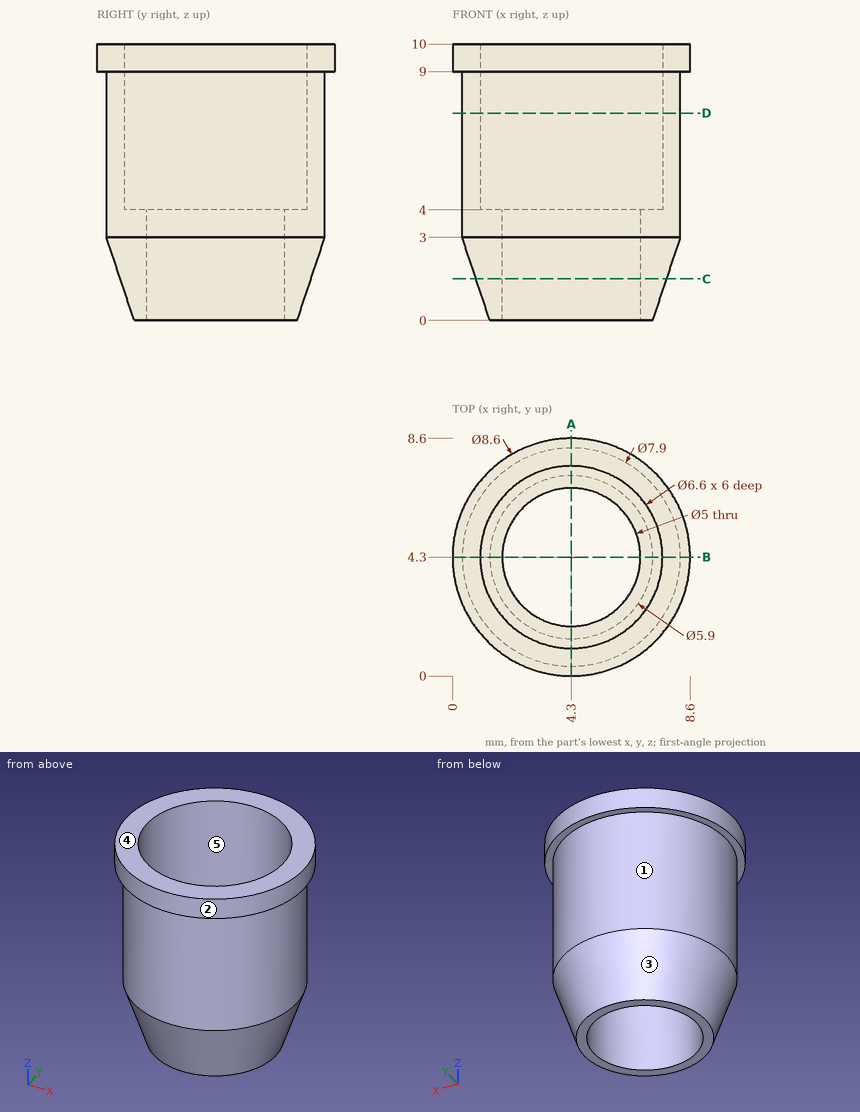
Print and shaded views of the part. All mm, measured from the part's lowest x, y and z. A direction names the side the tool comes from. Round coordinates to 2 decimals unless told otherwise and drop trailing zeros. Write each loop counter-clockwise with the first axis right and the second up, starting at its lowest first coordinate (ties: lowest second). Pieces come first, ordered by that corner, then holes. Notation, with made-up numbers: (-17.75, -26.75) -> (32.25, -26.75) arc R26 ccw to (32.25, -1.75) -> close; hole circle Ø1 at (-38.5, -33.75). An arc over 180 degrees is marked (long way). Return JSON: item names as keys, results as strings. Group by question number.
Q1. Mould opens along X. For the marked faces 3, 4 and 5 say: pulls with the +X half, pulls with the -X half, needs draft (parallel to the pull), parting line crosses it, or undercut.
Q2. Probe L1, parallel to Y at x = 4.3, z = 7.9; L2, parallel to Z at x = 5, y = 1.75; L3, parallel to X at y = 1.75, z = 7. List the from-to ranges inside material, lowest first. Write a range as [from, to].
Q3. Which spindle directions (+Z, -Z, +X, -X, +Y, -Y) get a long thin tool onto all of the face, cutting with end or side? Do the marked faces 1 and 2. Say none if no direction does.
Q4. Saw through at C-C on z = 1.5. Write the cut outline in (x, y).
Q5. Saw through at D-D on z = 7.5. Write the cut outline in (x, y), plus the area to 3 significant figures.
Q6. Saw through at A-A on x = 4.3. Write the cut outline in (y, z), plus the area to 3 significant figures.
Q7. Pin check, flat tips, straight feed: pin 1 (3 mm diameter, centred on y = 2.5, z = 5, fed in from +X); pin 2 (5 mm diameter, centred on x = 4.5, z = 1.5, fed in from +Y); pin 3 (1.5 mm diameter, centred on y = 3, z = 7, fed in from -X). Stop position of each tip, or through.
Answer:
{
 "1": {"face 3": "parting line crosses it", "face 4": "needs draft", "face 5": "undercut"},
 "2": {"L1": "[0.35, 1], [7.6, 8.25]", "L2": "[0, 4]", "L3": "[1.28, 2.21], [6.39, 7.32]"},
 "3": {"face 1": "-Z", "face 2": "+Z, -Z"},
 "4": {"outline": "circle Ø6.9 at (4.3, 4.3); hole circle Ø5 at (4.3, 4.3)"},
 "5": {"outline": "circle Ø7.9 at (4.3, 4.3); hole circle Ø6.6 at (4.3, 4.3)", "area": "14.8 mm2"},
 "6": {"outline": "(0, 9) -> (0.35, 9) -> (0.35, 3) -> (1.35, 0) -> (1.8, 0) -> (1.8, 4) -> (1, 4) -> (1, 10) -> (0, 10) -> close; (6.8, 0) -> (7.25, 0) -> (8.25, 3) -> (8.25, 9) -> (8.6, 9) -> (8.6, 10) -> (7.6, 10) -> (7.6, 4) -> (6.8, 4) -> close", "area": "17.1 mm2"},
 "7": {"pin 1": "x = 8.24", "pin 2": "y = 8.25", "pin 3": "x = 0.39"}
}
